Autodesk Inventor part; units mm, degrees
ref_plane "YZ Plane" through (0, 0, 0) normal (1, 0, 0) x (0, 1, 0)
ref_plane "XZ Plane" through (0, 0, 0) normal (0, 1, 0) x (-1, 0, 0)
ref_plane "XY Plane" through (0, 0, 0) normal (0, 0, 1) x (1, 0, 0)
sketch "Sketch1" plane through (0, 0, 0) normal (0, 0, 1) x (1, 0, 0)
  line L0 (-55.88, -28.575) -> (55.88, -28.575)
  line L1 (55.88, -28.575) -> (55.88, 28.575)
  line L2 (55.88, 28.575) -> (-55.88, 28.575)
  line L3 (-55.88, 28.575) -> (-55.88, -28.575)
  line L4 (-55.88, -28.575) -> (55.88, 28.575) construction
  line L5 (55.88, -28.575) -> (-55.88, 28.575) construction
  circle A0 centre (-52.07, 24.765) radius 1.4
  line L6 (-55.88, 0) -> (55.88, 0) construction
  line L7 (0, 28.575) -> (0, -28.575) construction
  circle A1 centre (-52.07, -24.765) radius 1.4
  circle A2 centre (-31.75, 24.765) radius 1.4
  circle A3 centre (31.75, 24.765) radius 1.4
  circle A4 centre (-31.75, -24.765) radius 1.4
  circle A5 centre (31.75, -24.765) radius 1.4
  circle A6 centre (50.8, 25.865) radius 0.99
  circle A7 centre (41.91, 24.765) radius 1.4
  circle A8 centre (41.91, -24.765) radius 1.4
  circle A9 centre (50.8, -2.71) radius 0.8
  point P0 (0, 0)
  dimension "d2" = 111.76
  dimension "d4" = 57.15
  dimension "d5" = 49.53
  dimension "d6" = 2.8
  dimension "d8" = 2.8
  dimension "d10" = 49.53
  dimension "d21" = 3.81
  dimension "d22" = 3.81
  dimension "d23" = 3.81
  dimension "d28" = 3.81
  dimension "d30" = 63.5
  dimension "d35" = 1.98
  dimension "d36" = 5.08
  dimension "d37" = 2.71
  dimension "d38" = 2.8
  dimension "d39" = 3.81
  dimension "d40" = 13.97
  dimension "d41" = 63.5
  dimension "d42" = 1.6
  dimension "d43" = 5.08
  dimension "d44" = 2.71
extrude "Extrusion1" add sketch "Sketch1" along normal blind 1.64 contours L3 L2 L1 L0 | A2 | A3 | A4 | A5
sketch "Sketch3" plane through (0, 0, 1.64) normal (0, 0, 1) x (1, 0, 0)
  circle A0 centre (26.67, -24.765) radius 1.4
  circle A1 centre (-26.67, -24.765) radius 1.4
  line L0 (55.88, 28.575) -> (-55.88, 28.575)
  line L1 (-21.67, -25.765) -> (21.67, -25.765)
  line L2 (21.67, -25.765) -> (21.67, 30.575)
  line L3 (21.67, 30.575) -> (-21.67, 30.575)
  line L4 (-21.67, 30.575) -> (-21.67, -25.765)
  line L5 (55.88, -28.575) -> (55.88, 28.575)
  line L6 (-55.88, 28.575) -> (-55.88, -28.575)
  point P0 (0, 0)
  dimension "d15" = 2
  dimension "d16" = 5
  dimension "d17" = 5
  dimension "d18" = 1
  dimension "d33" = 34.21
  dimension "d34" = 34.21
extrude "Extrusion3" [suppressed]
sketch "Sketch4" plane through (0, 0, 0) normal (0, 0, -1) x (-1, 0, 0)
  line L0 (-55.88, 28.575) -> (55.88, 28.575) construction
  line L1 (55.88, 28.575) -> (55.88, -28.575) construction
  line L2 (55.88, -28.575) -> (-55.88, -28.575) construction
  line L3 (-55.88, -28.575) -> (-55.88, 28.575) construction
  circle A0 centre (-41.91, -24.765) radius 1.4
  circle A1 centre (-41.91, 24.765) radius 1.4
  circle A2 centre (52.07, -24.765) radius 1.4
  circle A3 centre (52.07, 24.765) radius 1.4
  circle A4 centre (-50.8, 25.865) radius 0.99
  circle A5 centre (-50.8, -2.71) radius 0.8
  line L4 (55.88, -28.575) -> (-55.88, -28.575)
  line L5 (55.88, 28.575) -> (55.88, -28.575)
  line L6 (-55.88, 28.575) -> (55.88, 28.575)
  line L7 (-55.88, -28.575) -> (-55.88, 28.575)
  point P0 (0, 0)
sketch "Sketch5" plane through (0, 0, 1.64) normal (0, 0, 1) x (1, 0, 0)
  circle A0 centre (41.91, -24.765) radius 1.4
  circle A1 centre (41.91, 24.765) radius 1.4
  circle A2 centre (-52.07, -24.765) radius 1.4
  circle A3 centre (-52.07, 24.765) radius 1.4
  circle A4 centre (50.8, 25.865) radius 0.99
  circle A5 centre (50.8, -2.71) radius 0.8
  line L0 (-55.88, -28.575) -> (55.88, -28.575)
  line L1 (55.88, -28.575) -> (55.88, 28.575)
  line L2 (55.88, 28.575) -> (-55.88, 28.575)
  line L3 (-55.88, 28.575) -> (-55.88, -28.575)
  line L4 (55.88, -28.575) -> (-55.88, -28.575) construction
  line L5 (-55.88, -28.575) -> (-55.88, 28.575) construction
  line L6 (-55.88, 28.575) -> (55.88, 28.575) construction
  line L7 (55.88, 28.575) -> (55.88, -28.575) construction
  point P0 (0, 0)
properties part number "BetaBoard01" material "PCB(1)"
Verification items for the finished model (mm, model axes). Coordinates: 2 decimals unless noted, no trailing zeros. Write each loop counter-clockwise with the first axis right and the second up, starting at its lowest first coordinate (ties: lowest second). Pieces come first, ordered by that corner, then holes. Notation, with made-up numbers: M -5,34 L 43,34 A34 cw 43,66 Z; hole C 11,78.5 d7. An arc over 180 degrees is marked long. One line per question, with ' | ' between items.
1) Release check for a two-part mould opening along X. For faces 1 (the face through (43.245, 24.344, 0.809)), 2 (the face through (-1, 0, 0)) record: +X half, -X half, draft (parallel to the pull), parting line (faces both ways), or undercut.
Solutions:
face 1: undercut | face 2: draft
2) Material ranges on L1, parallel to Y at x = -52.07, z = 1 (3 decimals); L2, parallel to Y at x = 50.8, z = 1 (3 decimals); L3, parallel to X at y = -25, z = 0.95, recorded low to high.
Solutions:
L1: -28.575 to -26.165, -23.365 to 23.365, 26.165 to 28.575 | L2: -28.575 to -3.51, -1.91 to 24.875, 26.855 to 28.575 | L3: -55.88 to -53.45, -50.69 to 40.53, 43.29 to 55.88
3) Sectioned sample at A-A on x = 41.91. Record the cut outline in (y, z) (3 decimals).
Solutions:
outline: M -28.575,0 L -26.165,0 L -26.165,1.64 L -28.575,1.64 Z; M -23.365,0 L 23.365,0 L 23.365,1.64 L -23.365,1.64 Z; M 26.165,0 L 28.575,0 L 28.575,1.64 L 26.165,1.64 Z
